Geometry check sheet. Reference: the model listing, model coordinates, mm. A direction names the side the tool comes from. Round coordinates to 2 decimals unless told otherwise and drop trailing zeros. Order: outer loops, then holes, each group sorted by start corner. A loop starts at its lowest first (then second) coordinate and runs counter-clockwise, first axis right, second up. Notation, with made-up numbers: (41, -33.75) -> (75, -33.75) arc R18 ccw to (75, -7.75) -> close; hole circle Ø9 at (64, -27). An arc over 180 degrees is marked (long way). Use a Markdown table: item, result. Add a question column.
Item 1: Sectioned sample at B-B, the plane z = 75. Record the cut outline in (x, y).
Item 2: Gauge pin test, flat ends, axial feed: pin 1 Ø2.5 at (x, z) = (29, 56) entering from -Y; pin 2 Ø5 at (x, z) = (42.5, 75) entering from -Y; pin 3 Ø1 at (y, z) = (-1.5, 39) entering from -X; pin 4 Ø1 at (x, y) = (-4, -3) entering from +Z. Record the tip position at first contact, or that the pin passes through.
Item 3: Sectioned sample at D-D, the plane z = -75. Record the cut outline in (x, y), and give its area (3 significant figures).
Item 4: Sectioned sample at A-A, the plane x = 16.5. Record the cut outline in (y, z).
Item 5: Material ranges on probe 1 along X at (y, z) = (3.15, -59.5); probe 2 along Z at (x, y) = (42.5, -2.1); probe 3 along Z at (x, y) = (42.5, 3.3), recorded low to high. Write a range as [from, to].
Item 6: Mould release check, pull along X, two halves, no side actions. Record for faces 6 (the flat face through (23.5, 0, 14)), 7 (the flat face through (25, -2, 50.75)), 8 (the cylindrical face through (-48.786, 2.479, -58.131)): pulls with the +X half, pulls with the -X half, needs draft (parallel to the pull), parting line crosses it, or undercut.
Item 7: Set-up check for faces 1 (the flat face through (25.6, 1, 56.95)), 2 (the cylindrical face through (39.13, -1.54, -57.59)), 3 (the cylindrical face through (51.413, 0.056, -83.854)), 4 (the flat face through (-51.25, -2, -58)), 5 (the cylindrical face through (40.473, 2.479, 73.141)): record each of +Z, -Z, +X, -X, +Y, -Y from which the full face is reachable in a straight line by a thin tool's end or side.
Item 8: Sectioned sample at C-C, the plane x = 42.5. Record the cut outline in (y, z), and give its area (3 significant figures).
from build123d import *

# Parameters (mm, degrees)
SKETCH1_R                = 2.75
SKETCH1_R_2              = 2.25
BOSS_EXTRUDE1_DEPTH      = 4
BOSS_EXTRUDE1_DEPTH_BACK = 4
SKETCH2_R                = 4.25
CUT_EXTRUDE1_DEPTH       = 5


with BuildPart() as part:
    # Sketch1 → Boss-Extrude1 (new body, two sides)
    with BuildSketch(Plane(origin=(0, 0, 0), x_dir=(1, 0, 0), z_dir=(0, 1, 0))) as boss_extrude1_sk:
        with BuildLine():
            Line((-52.5, 81.188228139), (-52.5, 56))
            Line((-52.5, 56), (23.5, 56))
            Line((23.5, 56), (23.5, -85))
            Line((23.5, -85), (48.688228139, -85))
            ThreePointArc((48.688228139, -85), (51.38355787, -83.88355787), (52.5, -81.188228139))
            Line((52.5, -81.188228139), (52.5, 81.188228139))
            ThreePointArc((52.5, 81.188228139), (51.38355787, 83.88355787), (48.688228139, 85))
            Line((48.688228139, 85), (-48.688228139, 85))
            ThreePointArc((-48.688228139, 85), (-51.38355787, 83.88355787), (-52.5, 81.188228139))
        make_face()
        with Locations((42.5, -75)):
            Circle(SKETCH1_R, mode=Mode.SUBTRACT)
        with Locations((27, -55)):
            Circle(SKETCH1_R_2, mode=Mode.SUBTRACT)
        with Locations((-47, 59.5)):
            Circle(SKETCH1_R_2, mode=Mode.SUBTRACT)
        with Locations((-42.5, 75)):
            Circle(SKETCH1_R, mode=Mode.SUBTRACT)
        with Locations((16.5, 59.5)):
            Circle(SKETCH1_R_2, mode=Mode.SUBTRACT)
        with Locations((22.5, 75)):
            Circle(SKETCH1_R, mode=Mode.SUBTRACT)
        with Locations((42.5, 55)):
            Circle(SKETCH1_R, mode=Mode.SUBTRACT)
    extrude(amount=BOSS_EXTRUDE1_DEPTH)
    extrude(boss_extrude1_sk.sketch, amount=-BOSS_EXTRUDE1_DEPTH_BACK)

    # Sketch2 → Cut-Extrude1 (cut)
    with BuildSketch(Plane.XZ.offset(4)):
        with Locations((42.5, 75)):
            Circle(SKETCH2_R)
        with Locations((42.5, -55)):
            Circle(SKETCH2_R)
        with Locations((22.5, -75)):
            Circle(SKETCH2_R)
        with Locations((-42.5, -75)):
            Circle(SKETCH2_R)
        with BuildLine():
            Line((27, 59.25), (23.5, 59.25))
            Line((23.5, 59.25), (23.5, 50.75))
            Line((23.5, 50.75), (27, 50.75))
            ThreePointArc((27, 50.75), (31.25, 55), (27, 59.25))
        make_face()
        with BuildLine():
            Line((12.25, -59.5), (12.25, -56))
            Line((12.25, -56), (20.75, -56))
            Line((20.75, -56), (20.75, -59.5))
            ThreePointArc((20.75, -59.5), (16.5, -63.75), (12.25, -59.5))
        make_face()
        with BuildLine():
            Line((-51.25, -59.5), (-51.25, -56))
            Line((-51.25, -56), (-42.75, -56))
            Line((-42.75, -56), (-42.75, -59.5))
            ThreePointArc((-42.75, -59.5), (-47, -63.75), (-51.25, -59.5))
        make_face()
    extrude(amount=-CUT_EXTRUDE1_DEPTH, mode=Mode.SUBTRACT)


solid = part.part
Found:
| question | item | result |
|---|---|---|
| 1 | outline | (23.5, -4) -> (38.25, -4) -> (38.25, 1) -> (39.75, 1) -> (39.75, 4) -> (23.5, 4) -> close; (45.25, 1) -> (46.75, 1) -> (46.75, -4) -> (52.5, -4) -> (52.5, 4) -> (45.25, 4) -> close |
| 2 | pin 1 | stops at y = 1 |
| 2 | pin 2 | passes through |
| 2 | pin 3 | stops at x = 23.5 |
| 2 | pin 4 | stops at z = -56 |
| 3 | outline | (-52.5, -4) -> (-46.75, -4) -> (-46.75, 1) -> (-45.25, 1) -> (-45.25, 4) -> (-52.5, 4) -> close; (-39.75, 1) -> (-38.25, 1) -> (-38.25, -4) -> (18.25, -4) -> (18.25, 1) -> (19.75, 1) -> (19.75, 4) -> (-39.75, 4) -> close; (25.25, 1) -> (26.75, 1) -> (26.75, -4) -> (52.5, -4) -> (52.5, 4) -> (25.25, 4) -> close |
| 3 | area | 722 mm2 |
| 4 | outline | (-4, -85) -> (4, -85) -> (4, -61.75) -> (1, -61.75) -> (1, -63.75) -> (-4, -63.75) -> close; (1, -57.25) -> (4, -57.25) -> (4, -56) -> (1, -56) -> close |
| 5 | probe 1 | x = [-52.5, -49.25], [-44.75, 14.25], [18.75, 52.5] |
| 5 | probe 2 | z = [-85, -59.25], [-50.75, 70.75], [79.25, 85] |
| 5 | probe 3 | z = [-85, -57.75], [-52.25, 72.25], [77.75, 85] |
| 6 | face 6 | pulls with the -X half |
| 6 | face 7 | needs draft |
| 6 | face 8 | undercut |
| 7 | face 1 | -X, -Y |
| 7 | face 2 | -Y |
| 7 | face 3 | -Z, +X, +Y, -Y |
| 7 | face 4 | +Z, -Y |
| 7 | face 5 | +Y, -Y |
| 8 | outline | (-4, -85) -> (4, -85) -> (4, -57.75) -> (1, -57.75) -> (1, -59.25) -> (-4, -59.25) -> close; (-4, -50.75) -> (1, -50.75) -> (1, -52.25) -> (4, -52.25) -> (4, 72.25) -> (1, 72.25) -> (1, 70.75) -> (-4, 70.75) -> close; (-4, 79.25) -> (1, 79.25) -> (1, 77.75) -> (4, 77.75) -> (4, 85) -> (-4, 85) -> close |
| 8 | area | 1,240 mm2 |
